Source: CAD feature listing. Evaluate the final solid. Frame: model axes, mm. A direction names the side the tool comes from. Give positions to 0.01 mm unless a question says otherwise; leave off trailing zeros. Order: outer loops, then holes, each group sorted by start corner. A loop starts at its lowest first (then second) coordinate and runs counter-clockwise, first axis right, second up. Notation, with made-up numbers: (17, 32.25) -> (38, 32.25) arc R8 ccw to (38, 47.25) -> close; hole circle Ø10 at (23, 10). An arc over 180 degrees is marked (long way). Use CSV: the item, a comma, the result in double quotes.
```python
from build123d import *

# Parameters (mm, degrees)
F0_W     = 304.8
F0_H     = 203.2
F1_DEPTH = 3.175
F2_W     = 203.2
F2_H     = 127
F3_DEPTH = 25.4
F4_R     = 25.4


with BuildPart() as f1:
    # F0 (on Front) → F1 (new body)
    with BuildSketch(Plane.XZ):
        Rectangle(F0_W, F0_H)
    extrude(amount=F1_DEPTH)

    # F2 (on face) → F3 (cut)
    with BuildSketch(Plane.XZ.offset(3.175)):
        Rectangle(F2_W, F2_H)
    extrude(amount=-F3_DEPTH, mode=Mode.SUBTRACT)

    # F4
    f4_edges = [f1.edges().sort_by_distance(p)[0] for p in [
        (-101.6, -1.5875, 63.5),
        (-101.6, -1.5875, -63.5),
        (101.6, -1.5875, -63.5),
        (101.6, -1.5875, 63.5),
    ]]
    fillet(f4_edges, radius=F4_R)


solid = f1.part
```
1. Section query B-B on y = -1.4. Return loops of the section in (x, z), plus the area to 3 significant figures.
Answer below:
outline,"(-152.4, -101.6) -> (152.4, -101.6) -> (152.4, 101.6) -> (-152.4, 101.6) -> close; hole (-101.6, -38.1) arc R25.4 ccw to (-76.2, -63.5) -> (76.2, -63.5) arc R25.4 ccw to (101.6, -38.1) -> (101.6, 38.1) arc R25.4 ccw to (76.2, 63.5) -> (-76.2, 63.5) arc R25.4 ccw to (-101.6, 38.1) -> close"
area,"36,700 mm²"
2. Section query C-C on z = 22. Return loops of the section in (x, y) (3 decimals).
Answer below:
outline,"(-152.4, -3.175) -> (-101.6, -3.175) -> (-101.6, 0) -> (-152.4, 0) -> close; (101.6, -3.175) -> (152.4, -3.175) -> (152.4, 0) -> (101.6, 0) -> close"
3. Section query A-A on x = -6. Return loops of the section in (y, z) (3 decimals).
Answer below:
outline,"(-3.175, -101.6) -> (0, -101.6) -> (0, -63.5) -> (-3.175, -63.5) -> close; (-3.175, 63.5) -> (0, 63.5) -> (0, 101.6) -> (-3.175, 101.6) -> close"
4. Mould query, pull axis X, two halves, no side actions, for faces 1 (the flat face through (-2, 0, 69)), 2 (the cylindrical face through (93.96, -1.57, -56.26)). Classes: released by +X, released by -X, zero draft, split by the parting line, or undercut.
Answer below:
face 1,"zero draft"
face 2,"undercut"
5. Access query for faces 3 (the flat face through (-2, -3.175, 69)), 4 (the cylindrical face through (-93.96, -1.57, 56.26)). Directions: +Z, -Z, +X, -X, +Y, -Y. A direction counts if a zero-diameter tool reaches every point of the face in a straight line with its end or side. Return the directions, or none.
Answer below:
face 3,"+Z, -Z, +X, -X, -Y"
face 4,"+Y, -Y"
6. Ray query, line 1 along Z through (x, y) = (-1, -1); line 2 along X through (y, z) = (-0.3, 22); line 3 along X through (y, z) = (-2.5, 45). Return the intervals inside material, ascending.
Answer below:
line 1,"z = -101.6 to -63.5, 63.5 to 101.6"
line 2,"x = -152.4 to -101.6, 101.6 to 152.4"
line 3,"x = -152.4 to -100.64, 100.64 to 152.4"
